```python
from build123d import *

# Parameters (mm, degrees)
BOSS_EXTRUDE1_DEPTH = 6.35
FILLET1_R           = 6.35
SKETCH2_W           = 71.12
SKETCH2_H           = 11.43
CUT_EXTRUDE1_DEPTH  = 207.956858886
SKETCH3_R           = 0.635
CUT_EXTRUDE2_DEPTH  = 207.956858886
SKETCH6_OUTSIDE_W   = 361.165
SKETCH6_OUTSIDE_H   = 90.651
CUT_EXTRUDE4_DEPTH  = 207.956858886
FILLET3_R           = 6.35


with BuildPart() as part:
    # Sketch1 → Boss-Extrude1 (new body)
    with BuildSketch(Plane.XY):
        with BuildLine():
            add(Edge.make_bspline(
                [(36.979706214, 32.461234237), (-84.593483907, 33.006022806), (-204.294256369, 13.29140622)],
                knots=[1.565963281, 1.565963281, 1.565963281, 1.746596348, 1.746596348, 1.746596348], degree=2, weights=[1, 0.995924234, 1]))
            add(Edge.make_bspline(
                [(-204.294256369, 13.29140622), (-90.184781375, 5.397938815), (24.279187945, 3.948004614)],
                knots=[4.63926443, 4.63926443, 4.63926443, 4.706613661, 4.706613661, 4.706613661], degree=2, weights=[1, 0.999433064, 1]))
            add(Edge.make_bspline(
                [(24.279187945, 3.948004614), (64.56807699, 3.437658533), (103.433890649, 13.29140622)],
                knots=[4.698727851, 4.698727851, 4.698727851, 4.979307673, 4.979307673, 4.979307673], degree=2, weights=[1, 0.9901755, 1]))
            add(Edge.make_bspline(
                [(103.433890649, 13.29140622), (94.233757809, 22.223302177), (81.53716289, 25.9598127)],
                knots=[0.762399197, 0.762399197, 0.762399197, 1.263449558, 1.263449558, 1.263449558], degree=2, weights=[1, 0.968782356, 1]))
            add(Edge.make_bspline(
                [(81.53716289, 25.9598127), (59.792823381, 32.359005074), (36.979706214, 32.461234237)],
                knots=[1.263449558, 1.263449558, 1.263449558, 1.565963281, 1.565963281, 1.565963281], degree=2, weights=[1, 0.988582474, 1]))
        make_face()
    extrude(amount=BOSS_EXTRUDE1_DEPTH)

    # Fillet1
    fillet1_edges = [part.edges().sort_by_distance(p)[0] for p in [
        (103.433890649, 13.29140622, 3.175),
    ]]
    fillet(fillet1_edges, radius=FILLET1_R)

    # Sketch2 → Cut-Extrude1 (cut, through all)
    with BuildSketch(Plane(origin=(0, 0, 0), x_dir=(-1, 0, 0), z_dir=(0, 0, -1))):
        with Locations((46.047690277, 19.812)):
            Rectangle(SKETCH2_W, SKETCH2_H)
    extrude(amount=-CUT_EXTRUDE1_DEPTH, mode=Mode.SUBTRACT)

    # Sketch3 → Cut-Extrude2 (cut, through all)
    with BuildSketch(Plane.XY):
        with Locations((-1.343690277, 19.812)):
            Circle(SKETCH3_R)
        with Locations((-102.943690277, 19.812)):
            Circle(SKETCH3_R)
    extrude(amount=CUT_EXTRUDE2_DEPTH, mode=Mode.SUBTRACT)

    # Sketch6 outside → Cut-Extrude4 (cut, through all)
    with BuildSketch(Plane.XY):
        with Locations((-54.7605, 18.1995)):
            Rectangle(SKETCH6_OUTSIDE_W, SKETCH6_OUTSIDE_H)
        with BuildLine():
            add(Edge.make_bspline(
                [(-18.51330518, 28.052173793), (-112.124661574, 28.471660991), (-204.294256369, 13.29140622)],
                knots=[1.565963281, 1.565963281, 1.565963281, 1.746596348, 1.746596348, 1.746596348], degree=2, weights=[1, 0.995924234, 1]))
            add(Edge.make_bspline(
                [(-204.294256369, 13.29140622), (-116.429960623, 7.213436318), (-28.292704248, 6.096986983)],
                knots=[1.497671776, 1.497671776, 1.497671776, 1.565021007, 1.565021007, 1.565021007], degree=2, weights=[1, 0.999433064, 1]))
            add(Edge.make_bspline(
                [(-28.292704248, 6.096986983), (2.729740317, 5.704020501), (32.656416835, 13.29140622)],
                knots=[4.698727851, 4.698727851, 4.698727851, 4.979307673, 4.979307673, 4.979307673], degree=2, weights=[1, 0.9901755, 1]))
            add(Edge.make_bspline(
                [(32.656416835, 13.29140622), (25.572314548, 20.168966107), (15.79593646, 23.046079209)],
                knots=[0.762399197, 0.762399197, 0.762399197, 1.263449558, 1.263449558, 1.263449558], degree=2, weights=[1, 0.968782356, 1]))
            add(Edge.make_bspline(
                [(15.79593646, 23.046079209), (-0.947204961, 27.973457337), (-18.51330518, 28.052173793)],
                knots=[1.263449558, 1.263449558, 1.263449558, 1.565963281, 1.565963281, 1.565963281], degree=2, weights=[1, 0.988582474, 1]))
        make_face(mode=Mode.SUBTRACT)
    extrude(amount=CUT_EXTRUDE4_DEPTH, mode=Mode.SUBTRACT)

    # Fillet3
    fillet3_edges = [part.edges().sort_by_distance(p)[0] for p in [
        (32.656416835, 13.29140622, 3.175),
    ]]
    fillet(fillet3_edges, radius=FILLET3_R)


solid = part.part
```
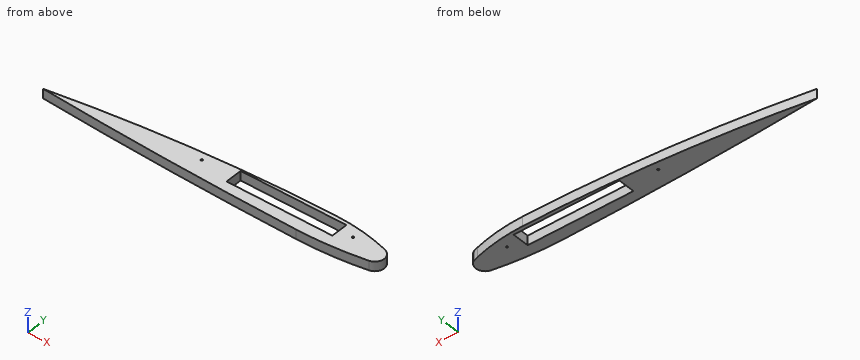
For this review, take the finished solid that the model builds, in its own axes (mm). Coordinates: 2 decimals unless noted, no trailing zeros.
(1) For pin 1 Ø3 at (x, z) = (-156, 2.5) entering from +Y; pin 2 Ø3 at (y, z) = (20, 4) entering from +X; pin 3 Ø2 at (x, y) = (-71.5, 24) entering from -Z, all flat-tipped, find the tip position at first contact; note any pin that passes through.
(2) Add section A-A on z = 2.5. Count the separate pieces of the cut face and the enclosed holes in it, then the cut area to 3 significant figures.
(3) Wall thickness on probe 1 along Y at (x, z) = (-19.5, 4.5); probe 2 along Y at (x, z) = (-76.5, 0.5); probe 3 along Y at (x, z) = (-132.5, 5.25): over which ranges is each line inside the solid? List them lowest first.
Answer sheet:
1. pin 1: stops at y = 20.34
1. pin 2: stops at x = 22.18
1. pin 3: passes through
2. separate pieces: 1
2. enclosed holes: 3
2. area: 2,610 mm2
3. probe 1: y = 6.15 to 14.1, 25.53 to 28.06
3. probe 2: y = 7.08 to 14.1, 25.53 to 26.8
3. probe 3: y = 9.16 to 22.72
